Part model, mm, in its own coordinate system. Face numbers are marked on the shaded views. A direction names the side the tool comes from. Coordinates: 2 decimals unless noted, no trailing zeros. Loops run counter-clockwise (first coordinate to the right, second up) from the corner with the lowest first, then second, coordinate; pieces in that order, holes last. Notation, with made-up numbers: M -2.75,56.25 L 56.25,56.25 A34 cw 56.25,89.25 Z; hole C 81,14 d10. An arc over 180 degrees is marked long. Use a Markdown table: item, result. Add a question column.
1) Pull direction X, two halves, no side cores. Call the marked faces 3, 4 and 5: released by +X, released by -X, zero draft, split by the parting line, or undercut.
2) Band-saw the part on C-C (z = -3). List the corners of the cut face in (x, y).
3) Pin check, flat tips, straight feed: pin 1 Ø3 at (x, y) = (-8.5, -2.5) entering from -Z; pin 2 Ø1.4 at (y, z) = (-5.5, 1.5) entering from +X; pin 3 Ø3.5 at (x, z) = (2, -0.5) entering from -Y; pin 4 Ø2 at (x, z) = (-4.5, 0) entering from -Y. Stop position of each tip, or through.
4) Band-saw the part on B-B (x = -4.5). List the corners of the cut face in (y, z).
5) Band-saw the part on D-D (y = -4.75). List the corners of the cut face in (x, z).
6) Wall check: probe 1 along Z at (x, y) = (-4.5, -1.05); probe 2 along Y at (x, z) = (5, 2.75); probe 3 along X at (y, z) = (-4.5, -1.5). Give the ranges that are in metal, low to high. Write a range as from..to.
7) Tool access for the marked faces 1 and 2: list every direction of +Z, -Z, +X, -X, +Y, -Y with a clear straight run to the whole face (end or side of a thin tool).
8) Band-saw the part on A-A (z = 0). List the corners of the cut face in (x, y), plus the area to 3 significant figures.
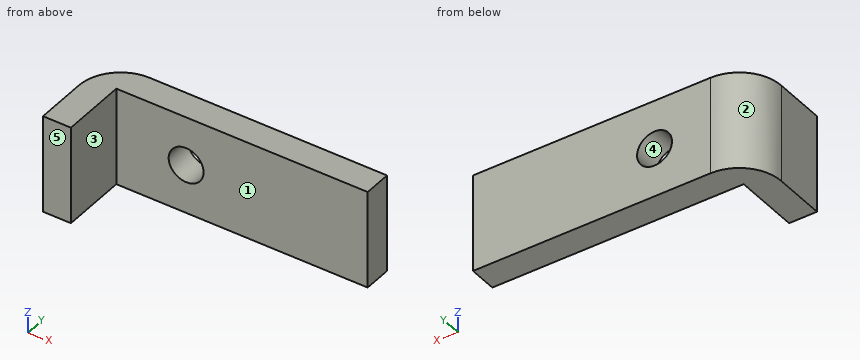
from build123d import *

# Parameters (mm, degrees)
EXTRUDE_1_DEPTH   = 3.5
HOLE_WIZARD_M31_D = 2.5


with BuildPart() as part:
    # Эскиз1 → Бобышка-Вытянуть1 (new, symmetric)
    with BuildSketch(Plane.XY):
        with BuildLine():
            Line((8.5, 0), (-8.5, 0))
            ThreePointArc((-8.5, 0), (-10.621320344, -0.878679656), (-11.5, -3))
            Line((-11.5, -3), (-11.5, -6.7))
            Line((-11.5, -6.7), (-9.5, -6.7))
            Line((-9.5, -6.7), (-9.5, -2))
            Line((-9.5, -2), (8.5, -2))
            Line((8.5, -2), (8.5, 0))
        make_face()
    extrude(amount=EXTRUDE_1_DEPTH, both=True)

    # Отверстие обработанное метчиком M31 (through all)
    with Locations(Plane(origin=(0, -2, 0), x_dir=(-1, 0, 0), z_dir=(0, -1, 0))):
        with Locations((4.5, 0)):
            Hole(HOLE_WIZARD_M31_D / 2)


solid = part.part
Entries:
| question | item | result |
|---|---|---|
| 1 | face 3 | released by +X |
| 1 | face 4 | undercut |
| 1 | face 5 | zero draft |
| 2 | outline | M -11.5,-6.7 L -9.5,-6.7 L -9.5,-2 L 8.5,-2 L 8.5,0 L -8.5,0 A3 ccw -11.5,-3 Z |
| 3 | pin 1 | z = -3.5 |
| 3 | pin 2 | x = -9.5 |
| 3 | pin 3 | y = -2 |
| 3 | pin 4 | through |
| 4 | outline | M -2,-3.5 L 0,-3.5 L 0,-1.25 L -2,-1.25 Z; M -2,1.25 L 0,1.25 L 0,3.5 L -2,3.5 Z |
| 5 | outline | M -11.5,-3.5 L -9.5,-3.5 L -9.5,3.5 L -11.5,3.5 Z |
| 6 | probe 1 | -3.5..-1.25, 1.25..3.5 |
| 6 | probe 2 | -2..0 |
| 6 | probe 3 | -11.5..-9.5 |
| 7 | face 1 | +Z, -Z, +X, -Y |
| 7 | face 2 | +Z, -Z, -X, +Y |
| 8 | outline | M -11.5,-6.7 L -9.5,-6.7 L -9.5,-2 L -5.75,-2 L -5.75,0 L -8.5,0 A3 ccw -11.5,-3 Z; M -3.25,-2 L 8.5,-2 L 8.5,0 L -3.25,0 Z |
| 8 | area | 42.5 mm2 |
